Build history of the part. All positions in model axes, mm. Face numbers are marked on the shaded views. A direction names the side the tool comes from. Coordinates: 2 decimals unless noted, no trailing zeros. Loops run counter-clockwise (first coordinate to the right, second up) from the corner with the lowest first, then second, coordinate; pieces in that order, holes last.
Item 1: Flat gauge pins, fed straight in: pin 1 (17 mm diameter, centred on y = 12.5, z = 35, fed in from -X); pin 2 (4 mm diameter, centred on y = 19.5, z = 40.5, fed in from +X); pin 3 (3.5 mm diameter, centred on x = -1, z = 24.5, fed in from +Y). Where does each tip first touch, or does it go through?
Item 2: Cut at D-D (z = -9.4). List the corners of the cut face in (x, y).
Item 3: Cut at B-B (x = -1). List the corners of the cut face in (y, z).
Item 4: 3-axis set-ups, long thin cutter, end or side, ignore diameter. For the marked faces 1, 2 and 3: which of +Z, -Z, +X, -X, +Y, -Y reach the whole face in a straight line?
Item 5: Drill centre lines: line 1 along X through (y, z) = (0.95, -9.4); line 2 along X through (y, z) = (9, 33); line 3 along Y through (x, z) = (-3.5, 40.5). Where is each one in solid material? Low to high.
Item 6: Cut at A-A (z = 40.5). List the corners of the cut face in (x, y), and give its area (3 significant figures).
Item 7: Cut at C-C (y = 1.5). List the corners of the cut face in (x, z), and give its area (3 significant figures).
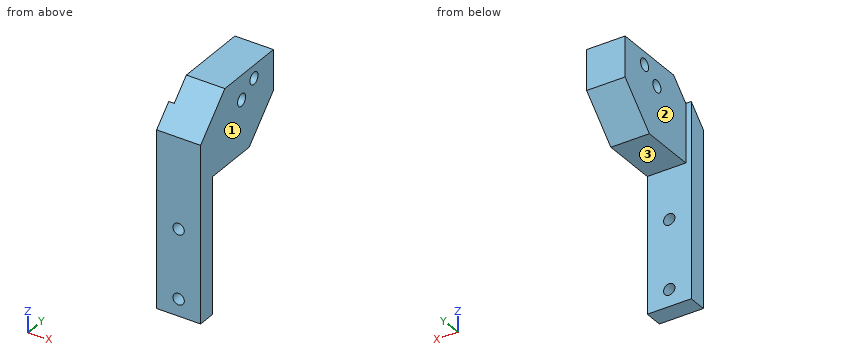
from build123d import *

# Parameters (mm, degrees)
SKETCH_1_W          = 12
SKETCH_1_H          = 28
SKETCH_1_R          = 1.55
EXTRUDE_1_DEPTH     = 2.5
SKETCH_2_W          = 12
SKETCH_2_H          = 5
EXTRUDE_2_DEPTH     = 30
SKETCH_3_W          = 10.5
SKETCH_3_H          = 21
EXTRUDE_3_DEPTH     = 25
CHAMFER_1_SIZE      = 10
SKETCH_4_R          = 1.65
CUT_EXTRUDE_1_DEPTH = 25
CHAMFER_2_SIZE      = 10


with BuildPart() as part:
    # 草图1 → 凸台-拉伸1 (new, symmetric)
    with BuildSketch(Plane(origin=(0, 0, 0), x_dir=(1, 0, 0), z_dir=(0, 1, 0))):
        Rectangle(SKETCH_1_W, SKETCH_1_H)
        with Locations(Location((0, 9.4, 0), (0, 0, 270))):
            Circle(SKETCH_1_R, mode=Mode.SUBTRACT)
        with Locations(Location((0, -9.4, 0), (0, 0, 90))):
            Circle(SKETCH_1_R, mode=Mode.SUBTRACT)
    extrude(amount=EXTRUDE_1_DEPTH, both=True)

    # 草图2 → 凸台-拉伸2 (add)
    with BuildSketch(Plane.XY.offset(14)):
        Rectangle(SKETCH_2_W, SKETCH_2_H)
    extrude(amount=EXTRUDE_2_DEPTH)

    # 草图3 → 凸台-拉伸3 (add)
    with BuildSketch(Plane(origin=(0, 2.5, 0), x_dir=(1, 0, 0), z_dir=(0, 1, 0))):
        with Locations((0.75, -33.5)):
            Rectangle(SKETCH_3_W, SKETCH_3_H)
    extrude(amount=EXTRUDE_3_DEPTH)

    # 倒角1
    chamfer_1_edges = [part.edges().sort_by_distance(p)[0] for p in [
        (0.75, 27.5, 23),
    ]]
    chamfer(chamfer_1_edges, length=CHAMFER_1_SIZE)

    # 草图4 → 切除-拉伸1 (cut)
    with BuildSketch(Plane.ZY.offset(4.5)):
        with Locations((40.5, 19.5)):
            Circle(SKETCH_4_R)
        with Locations((37.35, 14.393386641)):
            Circle(SKETCH_4_R)
    extrude(amount=-CUT_EXTRUDE_1_DEPTH, mode=Mode.SUBTRACT)

    # 倒角2
    chamfer_2_edges = [part.edges().sort_by_distance(p)[0] for p in [
        (0, -2.5, 44),
    ]]
    chamfer(chamfer_2_edges, length=CHAMFER_2_SIZE)


solid = part.part
Filled sheet:
1. pin 1: stops at x = -4.5
1. pin 2: stops at x = 6
1. pin 3: stops at y = 20.75
2. outline: (-6, -2.5) - (-1.55, -2.5) - (-1.55, 2.5) - (-6, 2.5) - close; (1.55, -2.5) - (6, -2.5) - (6, 2.5) - (1.55, 2.5) - close
3. outline: (-2.5, -14) - (2.5, -14) - (2.5, -10.58) - (-2.5, -10.58) - close; (-2.5, -8.22) - (2.5, -8.22) - (2.5, 8.22) - (-2.5, 8.22) - close; (-2.5, 10.58) - (2.5, 10.58) - (2.5, 23) - (17.5, 23) - (27.5, 33) - (27.5, 44) - (7.5, 44) - (-2.5, 34) - close; hole circle Ø3.3 at (14.39, 37.35); hole circle Ø3.3 at (19.5, 40.5)
4. face 1: +Z, -Z, +X, +Y, -Y
4. face 2: +Z, -Z, -X, +Y
4. face 3: -Z, +X, -X, +Y
5. line 1: x = -6 to -1.55, 1.55 to 6
5. line 2: x = -4.5 to 6
5. line 3: y = 4 to 17.85, 21.15 to 27.5
6. outline: (-4.5, 4) - (6, 4) - (6, 17.85) - (-4.5, 17.85) - close; (-4.5, 21.15) - (6, 21.15) - (6, 27.5) - (-4.5, 27.5) - close
6. area: 212 mm2
7. outline: (-6, -14) - (6, -14) - (6, 38) - (-6, 38) - close; hole circle Ø3.1 at (0, -9.4); hole circle Ø3.1 at (0, 9.4)
7. area: 609 mm2
